```python
from build123d import *

# Parameters (mm, degrees)
SKETCH1_W           = 400
SKETCH1_H           = 38
BOSS_EXTRUDE1_DEPTH = 48
SKETCH2_R           = 12
BOSS_EXTRUDE2_DEPTH = 25
BOSS_EXTRUDE3_START = 25
SKETCH3_R           = 12
BOSS_EXTRUDE3_DEPTH = 25
SKETCH6_R           = 12.5
CUT_EXTRUDE1_DEPTH  = 50


with BuildPart() as part:
    # Sketch1 → Boss-Extrude1 (new body)
    with BuildSketch(Plane(origin=(0, 0, 0), x_dir=(1, 0, 0), z_dir=(0, 1, 0))):
        Rectangle(SKETCH1_W, SKETCH1_H)
    extrude(amount=BOSS_EXTRUDE1_DEPTH)

    # Sketch2 → Boss-Extrude2 (add)
    with BuildSketch(Plane.XY.offset(19)):
        with Locations(Location((-176, 24, 0), (0, 0, 180))):
            Circle(SKETCH2_R)
    extrude(amount=BOSS_EXTRUDE2_DEPTH)

    # Sketch3 → Boss-Extrude3 (add)
    with BuildSketch(Plane(origin=(0, 0, -19), x_dir=(-1, 0, 0), z_dir=(0, 0, -1)).offset(BOSS_EXTRUDE3_START)):
        with Locations((176, 24)):
            Circle(SKETCH3_R)
    extrude(amount=-BOSS_EXTRUDE3_DEPTH)

    # Sketch6 → Cut-Extrude1 (cut)
    with BuildSketch(Plane(origin=(200, 0, 0), x_dir=(0, 0, -1), z_dir=(1, 0, 0))):
        with Locations((0, 24)):
            Circle(SKETCH6_R)
    extrude(amount=-CUT_EXTRUDE1_DEPTH, mode=Mode.SUBTRACT)


solid = part.part
```
The listing builds one solid part. Answer for the finished solid, in the listing's coordinates (mm). A direction names the side the tool comes from. Give positions to 0.01 mm unless a question says otherwise; leave off trailing zeros. Order: outer loops, then holes, each group sorted by start corner. A loop starts at its lowest first (then second) coordinate and runs counter-clockwise, first axis right, second up. Notation, with made-up numbers: (20, -34) -> (45, -34) arc R28 ccw to (45, -11) -> close; hole circle Ø7 at (25.25, 15.5). An arc over 180 degrees is marked (long way). Answer as CSV lines item,"result". Start each with the question number.
Q1. Which of the six approach directions +Z, -Z, +X, -X, +Y, -Y give full straight-line access (tool end or side, diameter ignored) to faces 1 (the cylindrical face through (-164.01, 24.53, -31.68)), 2 (the flat face through (150, 24, 0)), 3 (the cylindrical face through (-164.01, 23.47, 31.32))?
Q2. Find the intervals of material crossed by L1, parallel to Y at x = 173, z = 0; L2, parallel to Z at x = -94.5, y = 38; L3, parallel to X at y = 23.5, z = -10, in increasing order.
Q3. Determine the mould class of faces 4 (the flat face through (-3, 24, -19)), 5 (the flat face through (-3, 0, 0)), 6 (the cylindrical face through (175.35, 11.797, 2.71)) for opening direction Y: pulls with the +Y half, pulls with the -Y half, needs draft (parallel to the pull), parting line crosses it, or undercut.
Q4. Given pin 1 (1 mm diameter, centred on x = 124.5, y = 38, fed in from +Z); pin 2 (3 mm diameter, centred on x = 4.5, y = 13, fed in from -Z); pin 3 (4 mm diameter, centred on y = 33.5, z = 22.5, fed in from -X), each flat-ended and moving along its own axis, determine where each tip first touches the part or whether it passes through.
Q5. A cutting plane is placed at C-C (y = 24). Determine the outline of the cut face in (x, z), then the cut area to 4 significant figures.
Q6. A cutting plane is placed at B-B (z = -3.5). Determine the outline of the cut face in (x, y).
Q7. A cutting plane is placed at D-D (x = -6). Determine the outline of the cut face in (y, z).
Q8. A cutting plane is placed at A-A (x = -176). Determine the outline of the cut face in (y, z).
Results found:
1,face 1,"-Z"
1,face 2,"+X"
1,face 3,"+Z"
2,L1,"0 to 11.5, 36.5 to 48"
2,L2,"-19 to 19"
2,L3,"-200 to 150"
3,face 4,"needs draft"
3,face 5,"pulls with the -Y half"
3,face 6,"undercut"
4,pin 1,"z = 19"
4,pin 2,"z = -19"
4,pin 3,"x = -185.37"
5,outline,"(-200, -19) -> (-188, -19) -> (-188, -44) -> (-164, -44) -> (-164, -19) -> (200, -19) -> (200, -12.5) -> (150, -12.5) -> (150, 12.5) -> (200, 12.5) -> (200, 19) -> (-164, 19) -> (-164, 44) -> (-188, 44) -> (-188, 19) -> (-200, 19) -> close"
5,area,"15,150 mm2"
6,outline,"(-200, 0) -> (200, 0) -> (200, 12) -> (150, 12) -> (150, 36) -> (200, 36) -> (200, 48) -> (-200, 48) -> close"
7,outline,"(0, -19) -> (48, -19) -> (48, 19) -> (0, 19) -> close"
8,outline,"(0, -19) -> (12, -19) -> (12, -44) -> (36, -44) -> (36, -19) -> (48, -19) -> (48, 19) -> (36, 19) -> (36, 44) -> (12, 44) -> (12, 19) -> (0, 19) -> close"
